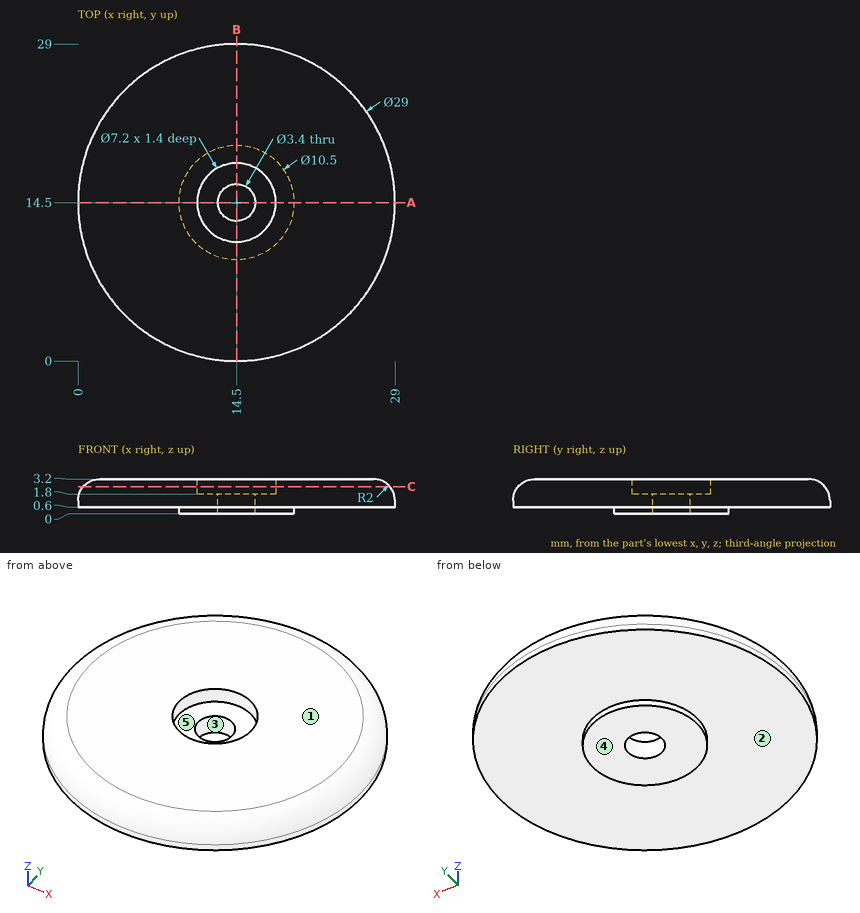
Input: dimensioned drawing with shaded views. Units: mm. Origin: part minimum x, y, z. A direction names the side the tool comes from. Round coordinates to 2 decimals unless told otherwise and drop trailing zeros. Loops run counter-clockwise (first coordinate to the right, second up) from the corner with the lowest first, then second, coordinate; pieces in that order, holes last. Notation, with made-up numbers: (64, -31) -> (95, -31) arc R10 cw to (95, -24) -> close; hole circle Ø11 at (16, -10.5). An arc over 180 degrees is marked (long way). Answer as a JSON object with one key per item and string values. Group by question number.
Q1. Section query A-A (y = 14.5). Output: boundary loops of the cut face in (x, z), plus the area to 3 significant figures.
Q2. Mould query, pull axis X, two halves, no side actions, for the marked faces 3, 4 and 5. Classes: pulls with the +X half, pulls with the -X half, needs draft (parallel to the pull), parting line crosses it, or undercut.
Q3. Access query for the marked faces 1 and 2. Directions: +Z, -Z, +X, -X, +Y, -Y. A direction counts if a zero-diameter tool reaches every point of the face in a straight line with its end or side. Return the directions, or none.
Q4. Contact query for flat-ended pins moving along their axis: P1, Ø1, axis at x = 17, z = 2, coming from the +Y side; P2, Ø2, axis at x = 14.5, y = 14.5, coming from the +Z side; P3, Ø1.5, axis at x = 16, z = 1, coming from the -Y side; P4, Ø1, axis at x = 6.5, z = 2.5, coming from the +Y side. Output: stop coordinate, or through.
Q5. Section query C-C (z = 2.5). Output: boundary loops of the cut face in (x, y), plus the area to 3 significant figures.
Q6. Ray query, line 1 (Y direction, x = 14.5, z = 1.3); line 2 (Z direction, x = 7, y = 10.5); line 3 (Y direction, x = 13, z = 2.45). Return the intervals inside material, ascending. Write a range as from..to.
Completed:
{
 "1": {"outline": "(0, 0.6) -> (9.25, 0.6) -> (9.25, 0) -> (12.8, 0) -> (12.8, 1.8) -> (10.9, 1.8) -> (10.9, 3.2) -> (2, 3.2) arc R2 ccw to (0, 1.2) -> close; (16.2, 0) -> (19.75, 0) -> (19.75, 0.6) -> (29, 0.6) -> (29, 1.2) arc R2 ccw to (27, 3.2) -> (18.1, 3.2) -> (18.1, 1.8) -> (16.2, 1.8) -> close", "area": "63.8 mm²"},
 "2": {"face 3": "undercut", "face 4": "needs draft", "face 5": "undercut"},
 "3": {"face 1": "+Z, +X, -X, +Y, -Y", "face 2": "-Z"},
 "4": {"P1": "y = 28.79", "P2": "through", "P3": "y = 0.02", "P4": "y = 26.54"},
 "5": {"outline": "circle Ø28.04 at (14.5, 14.5); hole circle Ø7.2 at (14.5, 14.5)", "area": "577 mm²"},
 "6": {"line 1": "0..12.8, 16.2..29", "line 2": "0.6..3.2", "line 3": "0.52..11.23, 17.77..28.48"}
}
